from build123d import *

# Parameters (mm, degrees)
SKETCH1_W           = 38
SKETCH1_H           = 18
SKETCH1_R           = 2.75
BOSS_EXTRUDE1_DEPTH = 2
FILLET1_R           = 1


with BuildPart() as part:
    # Sketch1 → Boss-Extrude1 (new, symmetric)
    with BuildSketch(Plane.XY):
        with Locations((19, 9)):
            Rectangle(SKETCH1_W, SKETCH1_H)
        with Locations((9, 9)):
            Circle(SKETCH1_R, mode=Mode.SUBTRACT)
        with Locations((29, 9)):
            Circle(SKETCH1_R, mode=Mode.SUBTRACT)
    extrude(amount=BOSS_EXTRUDE1_DEPTH, both=True)

    # Fillet1
    fillet1_edges = [part.edges().sort_by_distance(p)[0] for p in [
        (19, 18, 2),
        (0, 9, 2),
        (19, 0, 2),
        (38, 9, 2),
        (0, 0, 0),
        (0, 18, 0),
        (38, 18, 0),
        (38, 0, 0),
    ]]
    fillet(fillet1_edges, radius=FILLET1_R)


solid = part.part
Design review of the part built by this model. Coordinates are the model's own, in mm. Round coordinates to 2 decimals unless told otherwise and drop trailing zeros. Order: outer loops, then holes, each group sorted by start corner. A loop starts at its lowest first (then second) coordinate and runs counter-clockwise, first axis right, second up. Notation, with made-up numbers: M 7,76 L 22,76 A8 cw 22,83 Z; hole C 9,36.5 d6. An arc over 180 degrees is marked long. Answer as CSV lines item,"result". Start each with the question number.
1) Wall thickness on line 1 along Y through (x, z) = (9, -0.2); line 2 along X through (y, z) = (6.75, 0.75); line 3 along X through (y, z) = (10.5, 0.95): over which ranges is each line inside the solid? List them lowest first. Write a range as [from, to].
2) Add section B-B (z = -1.35). Give the boundary of the cut face in (x, y).
3) Add section A-A (y = 9). Give the boundary of the cut face in (x, z), then the cut area to 3 significant figures.
4) The part is to be moulded in two halves that separate along Y. For faces 1 (the face through (26.253, 9.121, -0.028)), 2 (the face through (37.699, 9.112, 1.715)), 3 (the face through (37.715, 17.699, -0.521)), 4 (the face through (19.252, 0.301, 1.715)), say which applies: +Y half, -Y half, draft (parallel to the pull), parting line (faces both ways), or undercut.
5) Add section C-C (x = 29). Give the boundary of the cut face in (y, z).
Resolved:
1,line 1,"[0, 6.25], [11.75, 18]"
1,line 2,"[0, 7.42], [10.58, 27.42], [30.58, 38]"
1,line 3,"[0, 6.7], [11.3, 26.7], [31.3, 38]"
2,outline,"M 0,1 A1 ccw 1,0 L 37,0 A1 ccw 38,1 L 38,17 A1 ccw 37,18 L 1,18 A1 ccw 0,17 Z; hole C 9,9 d5.5; hole C 29,9 d5.5"
3,outline,"M 0,-2 L 6.25,-2 L 6.25,2 L 1,2 A1 ccw 0,1 Z; M 11.75,-2 L 26.25,-2 L 26.25,2 L 11.75,2 Z; M 31.75,-2 L 38,-2 L 38,1 A1 ccw 37,2 L 31.75,2 Z"
3,area,"108 mm^2"
4,face 1,"undercut"
4,face 2,"draft"
4,face 3,"+Y half"
4,face 4,"-Y half"
5,outline,"M 0,-2 L 6.25,-2 L 6.25,2 L 1,2 A1 ccw 0,1 Z; M 11.75,-2 L 18,-2 L 18,1 A1 ccw 17,2 L 11.75,2 Z"
